from build123d import *


# Read off the part's stored shape, not the designer's step: Shell1
with BuildPart() as part:
    # Sketch1 → Revolve1 (revolve)
    with BuildSketch(Plane.XY, mode=Mode.PRIVATE) as revolve1_sk:
        with BuildLine():
            Line((0, 0), (55.850610629, 0))
            ThreePointArc((55.850610629, 0), (64.83086675, 3.719743879), (68.550610629, 12.7))
            Line((68.550610629, 12.7), (68.550610629, 135.537090781))
            ThreePointArc((68.550610629, 135.537090781), (67.07437947, 141.479902659), (62.988876295, 146.041145392))
            Line((62.988876295, 146.041145392), (36.426242146, 164.092378593))
            ThreePointArc((36.426242146, 164.092378593), (33.255344861, 167.632513451), (32.109591896, 172.244930881))
            Line((32.109591896, 172.244930881), (32.109591896, 182.693006016))
            Line((32.109591896, 182.693006016), (37.812538782, 182.693006016))
            Line((37.812538782, 182.693006016), (37.812538782, 191.889991998))
            Line((37.812538782, 191.889991998), (0, 191.889991998))
            Line((0, 191.889991998), (0, 0))
        make_face()
    revolve(revolve1_sk.sketch.rotate(Axis((0, 191.889991998, 0), (0, -1, 0)), 90), axis=Axis((0, 191.889991998, 0), (0, -1, 0)))

    # Shell1 outline → Shell1 (revolve, cut)
    with BuildSketch(Plane.XY):
        with BuildLine():
            Line((55.850610629, 0), (55.850610629, 2.54))
            ThreePointArc((55.850610629, 2.54), (63.034815526, 5.515795103), (66.010610629, 12.7))
            Line((66.010610629, 12.7), (66.010610629, 135.537090781))
            ThreePointArc((66.010610629, 135.537090781), (64.829625702, 140.291340284), (61.561223162, 143.94033447))
            Line((61.561223162, 143.94033447), (34.998589013, 161.991567671))
            ThreePointArc((34.998589013, 161.991567671), (31.010591093, 166.443951075), (29.569591896, 172.244930881))
            Line((29.569591896, 172.244930881), (29.569591896, 185.233006016))
            Line((29.569591896, 185.233006016), (35.272538782, 185.233006016))
            Line((35.272538782, 185.233006016), (35.272538782, 191.889991998))
            Line((35.272538782, 191.889991998), (0, 191.889991998))
            Line((0, 191.889991998), (0, 0))
            Line((0, 0), (55.850610629, 0))
        make_face()
    revolve(axis=Axis((0, 0, 0), (0, 1, 0)), mode=Mode.SUBTRACT)


solid = part.part
Work out the finished part from the listing and answer in its coordinate system (mm). A direction names the side the tool comes from. Coordinates: 2 decimals unless noted, no trailing zeros. Loops run counter-clockwise (first coordinate to the right, second up) from the corner with the lowest first, then second, coordinate; pieces in that order, holes last. Notation, with made-up numbers: M -16,79.25 L 31,79.25 A26 cw 31,107.25 Z; hole C 78.25,3.25 d2. An arc over 180 degrees is marked long. Answer in a Markdown table with one row per item. Add a question column.
1. Find section A-A, the plane y = 32.5. Write down the section's boundary in (x, z), then the cut area to 3 significant figures.
2. Find section B-B, the plane y = 157. Write down the section's boundary in (x, z), then the cut area to 3 significant figures.
3. Consider L1, parallel to X at y = 189.75, z = 0; L2, parallel to Z at x = -45.5, y = 36; L3, parallel to Z at x = -13, y = 103. Determine where each line is inside the solid, lowest interval first.
4. A tool of negligible diameter and unlimited length cuts with its end or side. For faces 1 (the cylindrical face through (-6.41, 178.83, 28.866)), 2 (the cylindrical face through (-44.321, 1.288, 33.984)), 3 (the conical face through (34.613, 161.115, -10.9)), 4 (the cylindrical face through (-7.646, 188.608, 34.434)), from which of +Z, -Z, +X, -X, +Y, -Y can it reach the whole face along a straight path? Write none if from no direction.
5. Flat-ended cylindrical pins translate along their axes: P1, Ø1.5, axis at x = -22, y = 74, coming from the -Z side; P2, Ø3, axis at y = 167, z = 19.5, coming from the -X side; P3, Ø5, axis at y = 79.5, z = 15, coming from the +X side. Find the tip coordinate at first contact, or state that the pin passes through.
6. The mould has two halves that part along Y. Classify faces 5 (the flat face through (8, 185.233, 29)), 6 (the cylindrical face through (23.008, 187.356, -30.007)), 7 (the cylindrical face through (-21.701, 177.542, -23.666)): pulls with the +Y half, pulls with the -Y half, needs draft (parallel to the pull), parting line crosses it, or undercut.
Reported:
| question | item | result |
|---|---|---|
| 1 | outline | C 0,0 d137.1; hole C 0,0 d132.02 |
| 1 | area | 1,070 mm^2 |
| 2 | outline | C 0,0 d93.73; hole C 0,0 d84.69 |
| 2 | area | 1,270 mm^2 |
| 3 | L1 | x = -37.81 to -35.27, 35.27 to 37.81 |
| 3 | L2 | z = -51.27 to -47.82, 47.82 to 51.27 |
| 3 | L3 | z = -67.31 to -64.72, 64.72 to 67.31 |
| 4 | face 1 | +Y, -Y |
| 4 | face 2 | -Y |
| 4 | face 3 | none |
| 4 | face 4 | +Y |
| 5 | P1 | stops at z = -65.17 |
| 5 | P2 | stops at x = -29.07 |
| 5 | P3 | stops at x = 67.4 |
| 6 | face 5 | pulls with the +Y half |
| 6 | face 6 | needs draft |
| 6 | face 7 | undercut |
